Drawing for the job (mm, zero at the part's lowest x, y, z). Round coordinates to 2 decimals unless told otherwise and drop trailing zeros. Loops run counter-clockwise (first coordinate to the right, second up) from the corner with the lowest first, then second, coordinate; pieces in that order, holes last. Notation, with made-up numbers: M -22.75,1.25 L 8.25,1.25 A10 cw 8.25,10.25 Z; hole C 27.25,39 d3. An arc over 180 degrees is marked long. Answer in a Markdown table with one row per item.
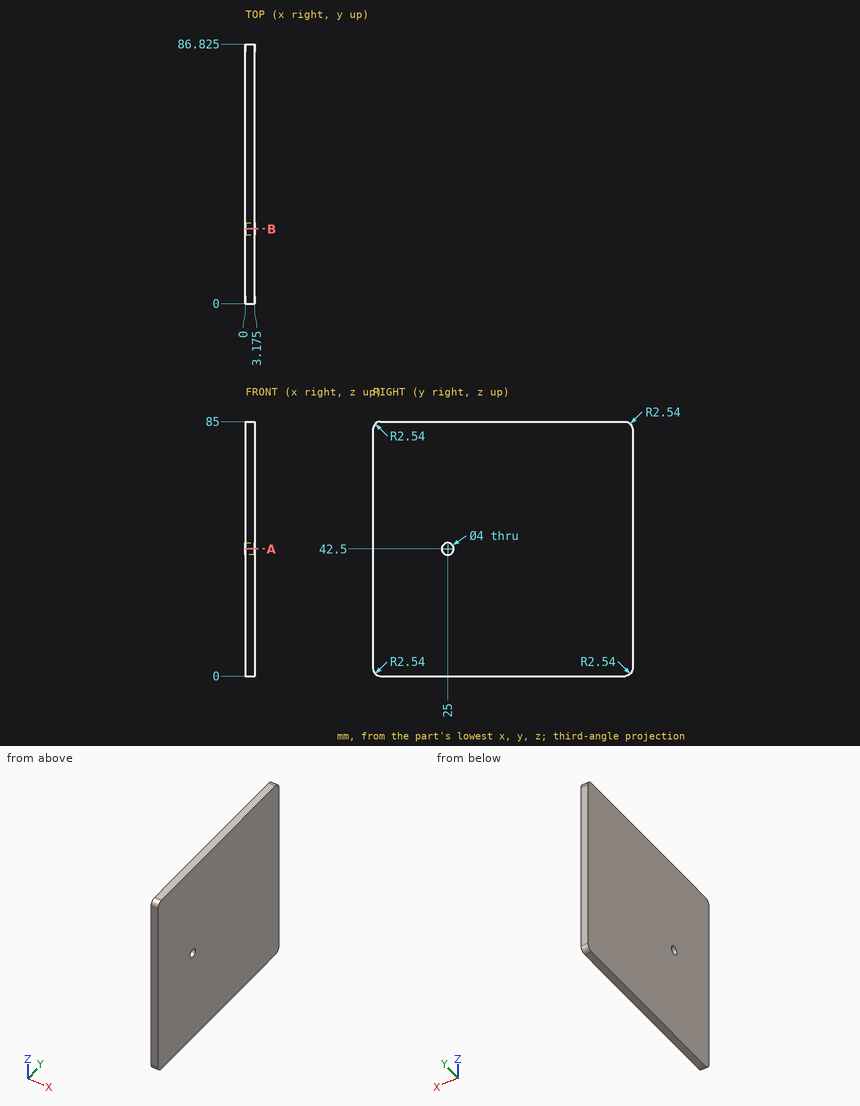
1. Pin check, flat tip, straight feed: pin 1 (2.5 mm diameter, centred on y = 25, z = 42.5, fed in from -X). Stop position of the tip, or through.
Verdict:
| item | result |
|---|---|
| pin 1 | passes through |
2. Wall check: probe 1 along Y at (x, z) = (1.15, 42.5) (3 decimals); probe 2 along Y at (x, z) = (1.15, 41) (3 decimals). Give the ranges that are in metal, low to high.
Verdict:
| item | result |
|---|---|
| probe 1 | y = 0 to 23, 27 to 86.825 |
| probe 2 | y = 0 to 23.677, 26.323 to 86.825 |
3. Saw through at B-B (y = 25). Write the cut outline in (x, z) (3 decimals), and give its area (3 significant figures).
Verdict:
| item | result |
|---|---|
| outline | M 0,0 L 3.175,0 L 3.175,40.5 L 0,40.5 Z; M 0,44.5 L 3.175,44.5 L 3.175,85 L 0,85 Z |
| area | 257 mm² |
4. Saw through at A-A (z = 42.5). Write the cut outline in (x, y) (3 decimals), and give its area (3 significant figures).
Verdict:
| item | result |
|---|---|
| outline | M 0,0 L 3.175,0 L 3.175,23 L 0,23 Z; M 0,27 L 3.175,27 L 3.175,86.825 L 0,86.825 Z |
| area | 263 mm² |
